For this review, take the finished solid that the model builds, in its own axes (mm). Face numbers are marked on the shaded views. A direction names the side the tool comes from. Give positions to 0.01 mm unless a question says otherwise; leave off trailing zeros. Order: outer loops, then holes, each group sorted by start corner. A loop starts at its lowest first (then second) coordinate and runs counter-clockwise, first axis right, second up. Notation, with made-up numbers: (-29, 19.5) - (9, 19.5) arc R26 ccw to (9, 47.5) - close; hole circle Ø11 at (-36, 89). An arc over 180 degrees is marked (long way). Put each result on its own line as item: value. Start each with the question number.
```python
from build123d import *

# Parameters (mm, degrees)
F6_W      = 65
F6_H      = 40
F6_R      = 6.5
F7_DEPTH  = 4
F8_DEPTH  = 0.6
F6_W_2    = 20
F6_H_2    = 18
F6_H_3    = 2
F9_DEPTH  = 9
F11_DEPTH = 18
F12_R     = 6.5
F13_SIZE  = 0.4


with BuildPart() as f7:
    # F6 (on Top) → F7 (new body)
    with BuildSketch(Plane.XY):
        with Locations((32.5, 20)):
            Rectangle(F6_W, F6_H)
        with Locations((8.5, 8.5)):
            Circle(F6_R, mode=Mode.SUBTRACT)
        with Locations((56.5, 8.5)):
            Circle(F6_R, mode=Mode.SUBTRACT)
        with Locations((8.5, 31.5)):
            Circle(F6_R, mode=Mode.SUBTRACT)
        Polygon((22.5, 30), (42.5, 30), (42.5, 28), (42.5, 10), (22.5, 10), (22.5, 28), align=None, mode=Mode.SUBTRACT)
        with Locations((56.5, 31.5)):
            Circle(F6_R, mode=Mode.SUBTRACT)
    extrude(amount=F7_DEPTH)

    # F6 (on Top) → F8 (join)
    with BuildSketch(Plane.XY):
        with Locations((8.5, 31.5)):
            Circle(F6_R)
        with Locations((8.5, 8.5)):
            Circle(F6_R)
        with Locations((56.5, 8.5)):
            Circle(F6_R)
        with Locations((56.5, 31.5)):
            Circle(F6_R)
    extrude(amount=F8_DEPTH)

    # F6 (on Top) → F9 (join)
    with BuildSketch(Plane.XY):
        with Locations((32.5, 19)):
            Rectangle(F6_W_2, F6_H_2)
        with Locations((32.5, 29)):
            Rectangle(F6_W_2, F6_H_3)
    extrude(amount=F9_DEPTH)

    # F10 (on face) → F11 (cut)
    with BuildSketch(Plane.XZ.offset(-10)):
        Polygon((26.1602540378, 4), (38.8397459622, 4), (37.5, 9), (27.5, 9), align=None)
    extrude(amount=-F11_DEPTH, mode=Mode.SUBTRACT)

    # F12
    f12_edges = [f7.edges().sort_by_distance(p)[0] for p in [
        (0, 0, 2),
        (0, 40, 2),
        (65, 0, 2),
        (65, 40, 2),
    ]]
    fillet(f12_edges, radius=F12_R)

    # F13
    f13_edges = [f7.edges().sort_by_distance(p)[0] for p in [
        (0, 20, 0),
        (1.903806, 38.096194, 0),
        (1.903806, 1.903806, 0),
        (32.5, 40, 0),
        (32.5, 0, 0),
        (63.096194, 38.096194, 0),
        (63.096194, 1.903806, 0),
        (65, 20, 0),
        (22.5, 20, 4),
        (22.5, 10, 6.5),
        (22.5, 20, 9),
        (22.5, 30, 6.5),
        (42.5, 20, 4),
        (42.5, 30, 6.5),
        (42.5, 20, 9),
        (42.5, 10, 6.5),
        (50, 8.5, 4),
        (50, 31.5, 4),
        (2, 8.5, 4),
        (2, 31.5, 4),
        (32.5, 0, 4),
        (0, 20, 4),
        (1.903806, 38.096194, 4),
        (1.903806, 1.903806, 4),
        (32.5, 40, 4),
        (63.096194, 38.096194, 4),
        (63.096194, 1.903806, 4),
        (65, 20, 4),
        (32.5, 30, 4),
        (40.669873, 10, 4),
        (24.330127, 10, 4),
    ]]
    chamfer(f13_edges, length=F13_SIZE)


solid = f7.part
```
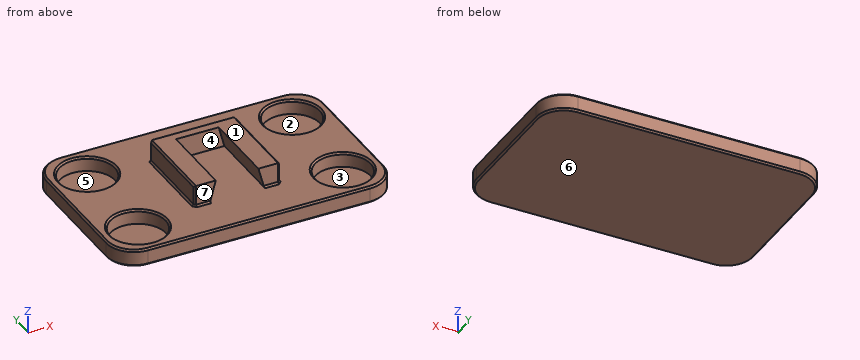
1. Add section A-A, the plane x = 8.5. Give the boundary of the cut face in (y, z), then the cut area to 3 significant figures.
2. The part is to be moulded in two halves that separate along Y. For the marked faces 1, 2, 3 and 4, say which applies: released by +Y, released by -Y, zero draft, split by the parting line, or undercut.
3. Add section C-C, the plane z = 2.5. Give the boundary of the cut face in (x, y).
4. Clearance check with flat-ended pins moving along their axes: pin 1 (10.5 mm diameter, centred on x = 8.5, y = 31.5, fed in from +Z); pin 2 (2.5 mm diameter, centred on x = 34.5, z = 5.5, fed in from -Y); pin 3 (10.5 mm diameter, centred on x = 6, y = 32, fed in from +Z). State where each tip first meets the part, or that it passes through.
5. Wall thickness on line 1 (Y direction, x = 56.5, z = 2.1); line 2 (X direction, y = 29.5, z = 2); line 3 (X direction, y = 28, z = 3.25): over which ranges is each line inside the solid? List them lowest first. Write a range as from..to.
6. Tool access review of the marked faces 5, 6 and 7: name each direction out of +Z, -Z, +X, -X, +Y, -Y from which nothing blocks a thin tool from reaching the whole face with its end or side.
7. Add section D-D, the plane x = 29. Give the boundary of the cut face in (y, z).
8. Add section B-B, the plane y = 18.5. Give the boundary of the cut face in (x, z).
Found:
1. outline: (0, 0.4) - (0.4, 0) - (39.6, 0) - (40, 0.4) - (40, 3.6) - (39.6, 4) - (38.4, 4) - (38, 3.6) - (38, 0.6) - (25, 0.6) - (25, 3.6) - (24.6, 4) - (15.4, 4) - (15, 3.6) - (15, 0.6) - (2, 0.6) - (2, 3.6) - (1.6, 4) - (0.4, 4) - (0, 3.6) - close
1. area: 71.0 mm^2
2. face 1: zero draft
2. face 2: undercut
2. face 3: undercut
2. face 4: released by -Y
3. outline: (0, 6.5) arc R6.5 ccw to (6.5, 0) - (58.5, 0) arc R6.5 ccw to (65, 6.5) - (65, 33.5) arc R6.5 ccw to (58.5, 40) - (6.5, 40) arc R6.5 ccw to (0, 33.5) - close; hole circle Ø13 at (8.5, 8.5); hole circle Ø13 at (8.5, 31.5); hole circle Ø13 at (56.5, 8.5); hole circle Ø13 at (56.5, 31.5)
4. pin 1: stops at z = 0.6
4. pin 2: stops at y = 28
4. pin 3: stops at z = 4
5. line 1: y = 0..2, 15..25, 38..40
5. line 2: x = 0..2.32, 14.68..50.32, 62.68..65
5. line 3: x = 0..3.02, 13.98..51.02, 61.98..65
6. face 5: +Z
6. face 6: -Z, +X, -X, +Y, -Y
6. face 7: +Z, +X, -X, -Y
7. outline: (0, 0.4) - (0.4, 0) - (39.6, 0) - (40, 0.4) - (40, 3.6) - (39.6, 4) - (30.4, 4) - (30, 4.4) - (30, 9) - (28, 9) - (28, 4) - (0.4, 4) - (0, 3.6) - close
8. outline: (0, 0.4) - (0.4, 0) - (64.6, 0) - (65, 0.4) - (65, 3.6) - (64.6, 4) - (42.9, 4) - (42.5, 4.4) - (42.5, 8.6) - (42.1, 9) - (37.5, 9) - (38.84, 4) - (26.16, 4) - (27.5, 9) - (22.9, 9) - (22.5, 8.6) - (22.5, 4.4) - (22.1, 4) - (0.4, 4) - (0, 3.6) - close
